Read the model definition and answer for the solid it produces. Units are mm, in the model's axes. Coordinates: 2 decimals unless noted, no trailing zeros. Loops run counter-clockwise (first coordinate to the right, second up) from the corner with the lowest first, then second, coordinate; pieces in that order, holes last. Notation, with made-up numbers: (-26.5, 18) - (25.5, 18) arc R18 ccw to (25.5, 37) - close; hole circle Ø5 at (-39.5, 43). An arc over 180 degrees is marked (long way). One line per question, with ' | ' between items. Start each with the question number.
```python
from build123d import *

# Parameters (mm, degrees)
F3_R = 1.5
F2_R = 5
F5_R = 1.5
F6_R = 0.5
F7_R = 10


with BuildPart() as f1:
    # F0 (on Right) → F1 (revolve)
    with BuildSketch(Plane.YZ):
        Polygon((-9.5, 0), (0, 0), (0, 25), (-2.5, 25), (-4.683943931, 12.5), align=None)
    revolve(axis=Axis((0, 0, 12.5), (0, 0, 1)))

    # F3 (on face) → F4 section 0
    with BuildSketch(Plane.XY.offset(25)):
        Circle(F3_R)
    # F2 (on face) → F4 section 1
    with BuildSketch(Plane(origin=(0, 0, 0), x_dir=(1, 0, 0), z_dir=(0, 0, -1))):
        Circle(F2_R)
    loft(mode=Mode.SUBTRACT)

    # F5
    f5_edges = [f1.edges().sort_by_distance(p)[0] for p in [
        (0, 9.5, 0),
    ]]
    fillet(f5_edges, radius=F5_R)

    # F6
    f6_edges = [f1.edges().sort_by_distance(p)[0] for p in [
        (-5, 0, 0),
        (0, 2.5, 25),
        (-1.5, 0, 25),
    ]]
    fillet(f6_edges, radius=F6_R)

    # F7
    f7_edges = [f1.edges().sort_by_distance(p)[0] for p in [
        (0, 4.683944, 12.5),
    ]]
    fillet(f7_edges, radius=F7_R)


solid = f1.part
```
1) Given pin 1 Ø6 at (y, z) = (-1, 16.5) entering from +X; pin 2 Ø6 at (x, y) = (-6, -6.5) entering from -Z; pin 3 Ø2 at (x, z) = (-3.5, 9) entering from -Y; pin 4 Ø2 at (x, z) = (-1.5, 14) entering from -Y, each flat-ended and moving along its own axis, determine where each tip first touches the part or whether it passes through.
2) The part is cut by section A-A on z = 8.5. Write down the section's boundary in (x, y).
3) Find the intervals of material crossed by line 1 along Z through (x, y) = (3.5, -5); line 2 along Y through (x, z) = (2, 1.75); line 3 along X through (y, z) = (-2.25, 2), in increasing order. Write a range as from..to.
4) The mould has two halves that part along Y. Classify faces 1 (the conical face through (-3.28, 0.14, 12.26)), 2 (the conical face through (1.069, -3.393, 18.946)), 3 (the flat face through (5.5, 1.1, 0)): released by +Y, released by -Y, zero draft, split by the parting line, or undercut.
5) The part is cut by section B-B on z = 13.75. Write down the section's boundary in (x, y) (3 decimals).
Answer below:
1) pin 1: x = 4.49 | pin 2: z = 0 | pin 3: y = -5.65 | pin 4: y = -4.48
2) outline: circle Ø12.45 at (0, 0); hole circle Ø7.62 at (0, 0)
3) line 1: 0..8.82 | line 2: -8.56..-4.31, 4.31..8.56 | line 3: -8.43..-4.15, 4.15..8.43
4) face 1: undercut | face 2: split by the parting line | face 3: zero draft
5) outline: circle Ø8.931 at (0, 0); hole circle Ø6.15 at (0, 0)
